The model under review builds one solid part; all positions refer to its coordinate system, in mm. A direction names the side the tool comes from. Coordinates: 2 decimals unless noted, no trailing zeros. Order: outer loops, then holes, each group sorted by start corner. A loop starts at its lowest first (then second) coordinate and runs counter-clockwise, first axis right, second up.
```python
from build123d import *

# Parameters (mm, degrees)
CROQUIS1_R              = 20
CROQUIS1_R_2            = 1
SALIENTE_EXTRUIR1_DEPTH = 5.5
CROQUIS2_W              = 5.5
CROQUIS2_H              = 21
SALIENTE_EXTRUIR2_DEPTH = 2.5
CROQUIS3_W              = 15.5
CROQUIS3_H              = 5.5
CROQUIS3_W_2            = 21
SALIENTE_EXTRUIR3_DEPTH = 2.5
CROQUIS4_W              = 5.5
CROQUIS4_H              = 21
SALIENTE_EXTRUIR4_DEPTH = 2.5
CROQUIS5_W              = 15.5
CROQUIS5_H              = 5.5
CROQUIS5_W_2            = 21
SALIENTE_EXTRUIR5_DEPTH = 2.5


with BuildPart() as part:
    # Croquis1 → Saliente-Extruir1 (new body)
    with BuildSketch(Plane.XY):
        Polygon((-47, 50), (-47, 31.5), (-50, 31.5), (-50, 10.5), (-47, 10.5), (-47, -10.5), (-50, -10.5), (-50, -31.5), (-47, -31.5), (-47, -50), (-31.5, -50), (-31.5, -47), (-10.5, -47), (-10.5, -50), (10.5, -50), (10.5, -47), (31.5, -47), (31.5, -50), (47, -50), (47, -31.5), (50, -31.5), (50, -10.5), (47, -10.5), (47, 10.5), (50, 10.5), (50, 31.5), (47, 31.5), (47, 50), (31.5, 50), (31.5, 47), (10.5, 47), (10.5, 50), (-10.5, 50), (-10.5, 47), (-31.5, 47), (-31.5, 50), align=None)
        Circle(CROQUIS1_R, mode=Mode.SUBTRACT)
        with Locations((25.684125329, 27.323537584)):
            Circle(CROQUIS1_R_2, mode=Mode.SUBTRACT)
        with Locations((25.684125329, -27.323537584)):
            Circle(CROQUIS1_R_2, mode=Mode.SUBTRACT)
        with Locations((-25.684125329, 27.323537584)):
            Circle(CROQUIS1_R_2, mode=Mode.SUBTRACT)
        with Locations((-25.684125329, -27.323537584)):
            Circle(CROQUIS1_R_2, mode=Mode.SUBTRACT)
    extrude(amount=SALIENTE_EXTRUIR1_DEPTH)

    # Croquis2 → Saliente-Extruir2 (add)
    with BuildSketch(Plane(origin=(50, 0, 0), x_dir=(0, 0, -1), z_dir=(1, 0, 0))):
        with Locations((-2.75, -21)):
            Rectangle(CROQUIS2_W, CROQUIS2_H)
        with Locations((-2.75, 21)):
            Rectangle(CROQUIS2_W, CROQUIS2_H)
    extrude(amount=SALIENTE_EXTRUIR2_DEPTH)

    # Croquis3 → Saliente-Extruir3 (add)
    with BuildSketch(Plane.XZ.offset(50)):
        with Locations((39.25, 2.75)):
            Rectangle(CROQUIS3_W, CROQUIS3_H)
        with Locations((0, 2.75)):
            Rectangle(CROQUIS3_W_2, CROQUIS3_H)
        with Locations((-39.25, 2.75)):
            Rectangle(CROQUIS3_W, CROQUIS3_H)
    extrude(amount=SALIENTE_EXTRUIR3_DEPTH)

    # Croquis4 → Saliente-Extruir4 (add)
    with BuildSketch(Plane.ZY.offset(50)):
        with Locations((2.75, -21)):
            Rectangle(CROQUIS4_W, CROQUIS4_H)
        with Locations((2.75, 21)):
            Rectangle(CROQUIS4_W, CROQUIS4_H)
    extrude(amount=SALIENTE_EXTRUIR4_DEPTH)

    # Croquis5 → Saliente-Extruir5 (add)
    with BuildSketch(Plane(origin=(0, 50, 0), x_dir=(1, 0, 0), z_dir=(0, 1, 0))):
        with Locations((-39.25, -2.75)):
            Rectangle(CROQUIS5_W, CROQUIS5_H)
        with Locations((0, -2.75)):
            Rectangle(CROQUIS5_W_2, CROQUIS5_H)
        with Locations((39.25, -2.75)):
            Rectangle(CROQUIS5_W, CROQUIS5_H)
    extrude(amount=SALIENTE_EXTRUIR5_DEPTH)


solid = part.part
```
(1) We need section A-A, the plane y = 0. Write out the cut boundary in (x, z).
A:
outline: (-47, 0) - (-20, 0) - (-20, 5.5) - (-47, 5.5) - close; (20, 0) - (47, 0) - (47, 5.5) - (20, 5.5) - close
(2) We need section D-D, the plane z = 3.25. Count the separate pieces of the cut face and the enclosed holes in it, and give its area (3 significant figures).
A:
separate pieces: 1
enclosed holes: 5
area: 8,600 mm2
(3) Machinability: for faces 5 (the face through (31.5, -50, 3)), 6 (the face through (-50, 31.5, 3)), 7 (the face through (10.5, 50, 3)), 8 (the face through (52.5, -21, 3)), 9 (the face through (47, 0, 3)), which of the approach directions +Z, -Z, +X, -X, +Y, -Y give a long, thin tool a straight path to every point of the face, cutting with its end or side? Answer none if there is none.
A:
face 5: +Z, -Z, -Y
face 6: +Z, -Z, -X, +Y
face 7: +Z, -Z, +Y
face 8: +Z, -Z, +X, +Y, -Y
face 9: +Z, -Z, +X
(4) Wall thickness on probe 1 along X at (y, z) = (38, 0.9); probe 2 along X at (y, z) = (-27, 4.8); probe 3 along Y at (x, z) = (13, 4.9): over which ranges is each line inside the solid? List them lowest first.
A:
probe 1: x = -47 to 47
probe 2: x = -52.5 to -26.63, -24.74 to 24.74, 26.63 to 52.5
probe 3: y = -47 to -15.2, 15.2 to 47
(5) Draft analysis for pull direction Y (two halves, no side actions). For faces 1 (the face through (-4.336, -19.524, 2.712)), 2 (the face through (52.5, 21, 3)), 3 (the face through (-21, -47, 3)), 4 (the face through (-50, -10.5, 3)), state which applies: released by +Y, released by -Y, zero draft, split by the parting line, or undercut.
A:
face 1: undercut
face 2: zero draft
face 3: released by -Y
face 4: undercut
(6) We need section C-C, the plane y = -38. Write out the cut boundary in (x, z), and give its area (3 significant figures).
A:
outline: (-47, 0) - (47, 0) - (47, 5.5) - (-47, 5.5) - close
area: 517 mm2
(7) We need section B-B, the plane x = 0. Write out the cut boundary in (y, z).
A:
outline: (-52.5, 0) - (-20, 0) - (-20, 5.5) - (-52.5, 5.5) - close; (20, 0) - (52.5, 0) - (52.5, 5.5) - (20, 5.5) - close
(8) For pin 1 Ø1.6 at (x, z) = (49.5, 2.5) entering from -Y; pin 2 Ø3 at (y, z) = (49, 2.5) entering from +X; pin 3 Ø3 at (x, z) = (-49, 2.5) entering from +Y, all flat-tipped, find the tip position at first contact; note any pin that passes through.
A:
pin 1: stops at y = -31.5
pin 2: stops at x = 47
pin 3: stops at y = 31.5
